Autodesk Inventor part; units mm, degrees
ref_plane "YZ Plane" through (0, 0, 0) normal (1, 0, 0) x (0, 1, 0)
ref_plane "XZ Plane" through (0, 0, 0) normal (0, 1, 0) x (-1, 0, 0)
ref_plane "XY Plane" through (0, 0, 0) normal (0, 0, 1) x (1, 0, 0)
sketch "Sketch1" plane through (0, 0, 0) normal (0, 1, 0) x (-1, 0, 0)
  circle A0 centre (0, 0) radius 20
  dimension "d0" = 40
extrude "Extrusion1" add sketch "Sketch1" along normal blind 6
sketch "Sketch2" plane through (0, 6, 0) normal (0, 1, 0) x (1, 0, 0)
  circle A0 centre (0, 0) radius 29.5
  dimension "d3" = 59
extrude "Extrusion2" add sketch "Sketch2" along normal blind 3
sketch "Sketch3" plane through (0, 6, 0) normal (0, -1, 0) x (1, 0, 0)
  circle A0 centre (0, 0) radius 29.5
  circle A1 centre (0, 0) radius 28
  dimension "d6" = 56
extrude "Extrusion3" add sketch "Sketch3" along normal blind 8.3
sketch "Sketch4" plane through (0, 9, 0) normal (0, 1, 0) x (1, 0, 0)
  circle A0 centre (0, 0) radius 14.5 construction
  line L0 (0, 0) -> (0, -14.5) construction
  point P0 (12.5574, 7.25)
  point P1 (-12.5574, 7.25)
  dimension "d9" = 29
  dimension "d12" = 360
hole "Hole1" at (0, 9, 14.5) at (12.5574, 9, -7.25) at (-12.5574, 9, -7.25) direction (0, -1, 0) diameter 4.3 end through all
chamfer "Chamfer1" distance 3 angle 45 1 edges at (20, 6, 0)
sketch "Sketch5" plane through (0, 9, 0) normal (0, 1, 0) x (1, 0, 0)
  circle A0 centre (0, -14.5) radius 2.15
  circle A1 centre (-12.5574, 7.25) radius 2.15
  circle A2 centre (12.5574, 7.25) radius 2.15
  circle A3 centre (0, -14.5) radius 4.25
  circle A4 centre (-12.5574, 7.25) radius 4.25
  circle A5 centre (12.5574, 7.25) radius 4.25
  point P0 (0, 0)
  dimension "d24" = 8.5
  dimension "d25" = 8.5
  dimension "d26" = 8.5
extrude "Extrusion4" cut sketch "Sketch5" against normal blind 5
equation "\"d25\" = d24"
equation "\"d26\" = d24"
properties part number "Arm - slew column C"
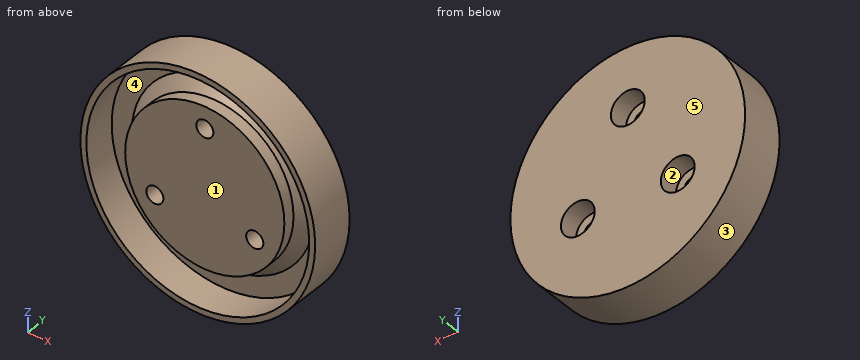
Geometry check sheet. Reference: the model listing, model coordinates, mm. Face numbers are marked on the shaded views. A direction names the side the tool comes from. Give positions to 0.01 mm unless a question says otherwise; leave off trailing zeros. Order: outer loops, then holes, each group sorted by start corner. A loop starts at its lowest first (then second) coordinate and runs counter-clockwise, first axis right, second up. Notation, with made-up numbers: (30, 31.25) - (35, 31.25) arc R8 ccw to (35, 39.25) - close; hole circle Ø1 at (66.5, 28). An arc over 180 degrees is marked (long way). Use one line per item in the form item = value.
1) Access from +Z, -Z, +X, -X, +Y, -Y to the whole of each face (thin tool, end or side, straight path). Record for the marked faces 1 and 2.
Working result:
face_1 = -Y
face_2 = +Y
2) Sectioned sample at B-B (z = 0). Record the boundary of the cut face in (x, y), and give its area (3 significant figures).
Working result:
outline = (-29.5, -2.3) - (-28, -2.3) - (-28, 6) - (-23, 6) - (-20, 3) - (-20, 0) - (20, 0) - (20, 3) - (23, 6) - (28, 6) - (28, -2.3) - (29.5, -2.3) - (29.5, 9) - (-29.5, 9) - close
area = 451 mm^2
3) Depth check by flat-ended pin: pin 1 Ø7.5 at (x, z) = (0, 14.5) entering from -Y; pin 2 Ø4 at (x, z) = (0, 14.5) entering from +Y; pin 3 Ø2 at (y, z) = (3.5, 6.5) entering from -X; pin 4 Ø5 at (x, z) = (12.56, -7.25) entering from +Y. Enter the tip coordinate at first touch or a pass-through.
Working result:
pin_1 = 0
pin_2 = through
pin_3 = -28.98
pin_4 = 4
4) Draft check along X on the marked faces 3, 4 and 5. Enter one of: released by +X, released by -X, zero draft, split by the parting line, or undercut.
Working result:
face_3 = split by the parting line
face_4 = undercut
face_5 = zero draft
5) Sectioned sample at A-A (x = 0). Record the boundary of the cut face in (y, z), and give its area (3 significant figures).
Working result:
outline = (-2.3, -29.5) - (9, -29.5) - (9, 10.25) - (4, 10.25) - (4, 12.35) - (0, 12.35) - (0, -20) - (3, -20) - (6, -23) - (6, -28) - (-2.3, -28) - close; (-2.3, 28) - (6, 28) - (6, 23) - (3, 20) - (0, 20) - (0, 16.65) - (4, 16.65) - (4, 18.75) - (9, 18.75) - (9, 29.5) - (-2.3, 29.5) - close
area = 391 mm^2
6) Material ranges on probe 1 along Z at (x, y) = (0, 1.5); probe 2 along Z at (x, y) = (-6, 3); probe 3 along X at (y, z) = (0.75, -9), recorded low to high. Write a range as from..to.
Working result:
probe_1 = -29.5..-28, -20..12.35, 16.65..20, 28..29.5
probe_2 = -28.88..-27.35, -19.08..19.08, 27.35..28.88
probe_3 = -28.09..-26.51, -17.86..-13.81, -11.31..11.31, 13.81..17.86, 26.51..28.09
7) Sectioned sample at C-C (y = -1). Record the boundary of the cut face in (x, z).
Working result:
outline = circle Ø59 at (0, 0); hole circle Ø56 at (0, 0)
8) Sectioned sample at D-D (z = -7.25). Count the separate pieces of the cut face and the enclosed holes in it, and give its area (3 significant figures).
Working result:
separate_pieces = 3
enclosed_holes = 0
area = 311 mm^2
